Can you work these out from the model? Positions are in its coordinate system, mm. Face numbers are marked on the shaded views. A direction names the side the tool comes from. Round coordinates to 2 decimals unless told otherwise and drop trailing zeros. Order: outer loops, then holes, each group sorted by start corner. A loop starts at its lowest first (then second) coordinate and runs counter-clockwise, first axis right, second up. Notation, with made-up numbers: M -22.5,25 L 19.5,25 A10 cw 19.5,37 Z; hole C 79.25,4.5 d7. An arc over 180 degrees is marked long. Answer as a JSON object with one key per item and string values. Group by question number.
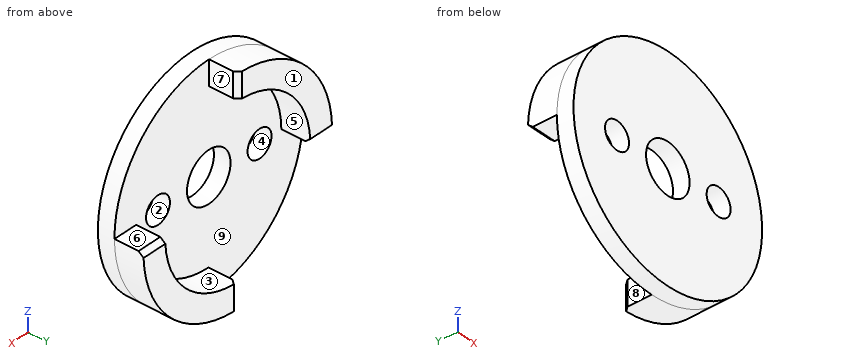
```python
from build123d import *
from OCP.BRepFilletAPI import BRepFilletAPI_MakeChamfer

# Parameters (mm, degrees)
SKETCH_1_R      = 13
SKETCH_1_R_2    = 1.65
SKETCH_1_R_3    = 3
EXTRUDE_1_DEPTH = 2
EXTRUDE_2_DEPTH = 3.5
CHAMFER_1_SIZE  = 0.5
CHAMFER_1_SIZE2 = 0.595876796


with BuildPart() as part:
    # 草图1 → 凸台-拉伸1 (new body)
    with BuildSketch(Plane(origin=(0, 0, 0), x_dir=(1, 0, 0), z_dir=(0, 1, 0))):
        with Locations(Location((0, 0, 0), (0, 0, 270))):
            Circle(SKETCH_1_R)
        with Locations(Location((7, 0, 0), (0, 0, 270))):
            Circle(SKETCH_1_R_2, mode=Mode.SUBTRACT)
        with Locations(Location((-7, 0, 0), (0, 0, 270))):
            Circle(SKETCH_1_R_2, mode=Mode.SUBTRACT)
        with Locations(Location((0, 0, 0), (0, 0, 270))):
            Circle(SKETCH_1_R_3, mode=Mode.SUBTRACT)
    extrude(amount=EXTRUDE_1_DEPTH)

    # 草图2 → 凸台-拉伸2 (add)
    with BuildSketch(Plane(origin=(0, 2, 0), x_dir=(1, 0, 0), z_dir=(0, 1, 0))):
        with BuildLine():
            ThreePointArc((12.999903846, 0.05), (9.192388155, 9.192388155), (0.05, 12.999903846))
            Line((0.05, 12.999903846), (0.05, 9.999874999))
            ThreePointArc((0.05, 9.999874999), (7.071067812, 7.071067812), (9.999874999, 0.05))
            Line((9.999874999, 0.05), (12.999903846, 0.05))
        make_face()
        with BuildLine():
            Line((-9.999874999, -0.05), (-12.999903846, -0.05))
            ThreePointArc((-12.999903846, -0.05), (-9.192388155, -9.192388155), (-0.05, -12.999903846))
            Line((-0.05, -12.999903846), (-0.05, -9.999874999))
            ThreePointArc((-0.05, -9.999874999), (-7.071067812, -7.071067812), (-9.999874999, -0.05))
        make_face()
    extrude(amount=EXTRUDE_2_DEPTH)

    # 倒角1: one chamfer whose edges measure the first distance from different faces: ONE call of the kernel's chamfer builder (chamfer() names one face for all edges)
    chamfer_1_edges_1 = [part.edges().sort_by_distance(p)[0] for p in [
        (11.499889423, 5.5, -0.05),
        (0.05, 5.5, -11.499889423),
    ]]
    chamfer_1_side_1 = [part.faces().sort_by_distance(p)[0] for p in [
        (7.371553631, 5.5, -7.371553631),
    ]]
    chamfer_1_edges_2 = [part.edges().sort_by_distance(p)[0] for p in [
        (-11.499889423, 5.5, 0.05),
        (-0.05, 5.5, 11.499889423),
    ]]
    chamfer_1_side_2 = [part.faces().sort_by_distance(p)[0] for p in [
        (-7.371553631, 5.5, 7.371553631),
    ]]
    chamfer_1 = BRepFilletAPI_MakeChamfer(part.part.solid().wrapped)
    for e in chamfer_1_edges_1:
        chamfer_1.Add(CHAMFER_1_SIZE, CHAMFER_1_SIZE2, e.wrapped, chamfer_1_side_1[0].wrapped)  # the first distance lies on this face
    for e in chamfer_1_edges_2:
        chamfer_1.Add(CHAMFER_1_SIZE, CHAMFER_1_SIZE2, e.wrapped, chamfer_1_side_2[0].wrapped)  # the first distance lies on this face
    add(Compound.cast(chamfer_1.Shape()), mode=Mode.REPLACE)


solid = part.part
```
1) We'd pull the mould along X, two halves only. Please class the marked faces 1, 2, 3 and 4: +X half, -X half, draft (parallel to the pull), parting line (faces both ways), or undercut.
2) If we section it at C-C on z = 7: Write out the boundary of the cut face in (x, y), plus the area to 3 significant figures.
3) If we section it at A-A on y = 3.65: Write out the boundary of the cut face in (x, z).
4) If we section it at D-D on y = 1.4: Write out the boundary of the cut face in (x, z).
5) Which directions (+Z, -Z, +X, -X, +Y, -Y) give clear straight access to the entire face, cutting with the end or side of a thin tool? Please do the marked faces 5, 6, 7, 8 and 9.
6) For pin 1 (1.5 mm diameter, centred on y = 3.5, z = -11.5, fed in from -X); pin 2 (9.5 mm diameter, centred on x = 0, z = 0, fed in from +Y); pin 3 (2 mm diameter, centred on y = 0.5, z = 7, fed in from +X); pin 4 (3 mm diameter, centred on x = 7, z = 0, fed in from -Y), each with a flat end and sliding along its axis, tell me the tip position at first contact or that it passes through.
7) If we section it at B-B on x = -2: Write out the boundary of the cut face in (y, z).
8) I need wall thicknesses on line 1 along X through (y, z) = (0.75, 0); line 2 along X through (y, z) = (1.45, 1); line 3 along Y through (x, z) = (-2.75, 5.75). Which ranges of each line are inside material? Lowest first, please.
Findings:
{
 "1": {"face 1": "draft", "face 2": "undercut", "face 3": "-X half", "face 4": "undercut"},
 "2": {"outline": "M -10.95,0 L 10.95,0 L 10.95,2 L -7.14,2 L -7.14,5.5 L -10.95,5.5 Z", "area": "57.2 mm^2"},
 "3": {"outline": "M -13,0.05 L -10,0.05 A10 cw -0.05,10 L -0.05,13 A13 ccw Z; M 0.05,-13 A13 ccw 13,-0.05 L 10,-0.05 A10 cw 0.05,-10 Z"},
 "4": {"outline": "C 0,0 d26; hole C -7,0 d3.3; hole C 0,0 d6; hole C 7,0 d3.3"},
 "5": {"face 5": "-Z, +X, +Y", "face 6": "+Z, +X, -X, +Y", "face 7": "+Z, -Z, +X, +Y", "face 8": "+Z, -Z, -X, +Y", "face 9": "+Y"},
 "6": {"pin 1": "stops at x = 0.05", "pin 2": "stops at y = 2", "pin 3": "stops at x = 11.53", "pin 4": "passes through"},
 "7": {"outline": "M 0,-12.85 L 2,-12.85 L 2,-2.24 L 0,-2.24 Z; M 0,2.24 L 2,2.24 L 2,9.8 L 5.5,9.8 L 5.5,12.85 L 0,12.85 Z"},
 "8": {"line 1": "x = -13 to -8.65, -5.35 to -3, 3 to 5.35, 8.65 to 13", "line 2": "x = -12.96 to -8.31, -5.69 to -2.83, 2.83 to 5.69, 8.31 to 12.96", "line 3": "y = 0 to 2"}
}
